Geometry check sheet. Reference: drawing and pictorial views, mm from the part's lowest x, y, z. A direction names the side the tool comes from. Coordinates: 2 decimals unless noted, no trailing zeros. Loops run counter-clockwise (first coordinate to the right, second up) from the corner with the lowest first, then second, coordinate; pieces in that order, holes last. Notation, with made-up numbers: (60, 58.25) - (95, 58.25) arc R30 cw to (95, 83.25) - close; hole circle Ø4 at (12, 48.25). An arc over 180 degrees is marked (long way). One line per item, written item: value.
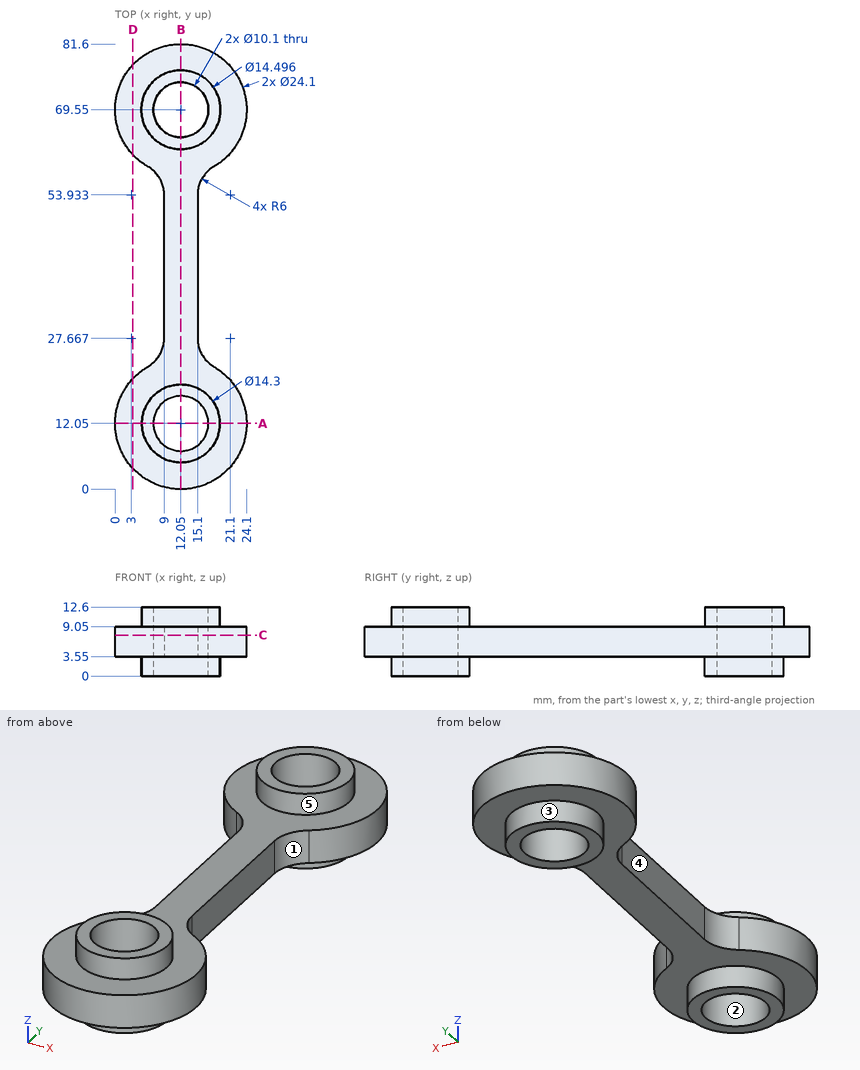
(1) Access from +Z, -Z, +X, -X, +Y, -Y to the whole of each face (thin tool, end or side, straight path). Record for the marked faces 1, 2, 3, 4 and 5.
Reply:
face 1: +Z, -Z, +X
face 2: +Z, -Z
face 3: -Z
face 4: +Z, -Z, -X
face 5: +Z
(2) Cross-section at B-B on x = 12.05. Record the cut outline in (y, z), and give its area (3 significant figures).
Reply:
outline: (0, 3.55) - (4.9, 3.55) - (4.9, 0) - (7, 0) - (7, 12.6) - (4.9, 12.6) - (4.9, 9.05) - (0, 9.05) - close; (17.1, 0) - (19.2, 0) - (19.2, 3.55) - (62.3, 3.55) - (62.3, 0) - (64.5, 0) - (64.5, 12.6) - (62.3, 12.6) - (62.3, 9.05) - (19.2, 9.05) - (19.2, 12.6) - (17.1, 12.6) - close; (74.6, 0) - (76.8, 0) - (76.8, 3.55) - (81.6, 3.55) - (81.6, 9.05) - (76.8, 9.05) - (76.8, 12.6) - (74.6, 12.6) - close
area: 399 mm2
(3) Cross-section at C-C on z = 7.5. Record the cut outline in (x, y), and give its area (3 significant figures).
Reply:
outline: (6.01, 22.48) arc R12.05 ccw (long way) to (18.09, 22.48) arc R6 cw to (15.1, 27.67) - (15.1, 53.93) arc R6 cw to (18.09, 59.12) arc R12.05 ccw (long way) to (6.01, 59.12) arc R6 cw to (9, 53.93) - (9, 27.67) arc R6 cw to start; hole circle Ø10.1 at (12.05, 12.05); hole circle Ø10.1 at (12.05, 69.55)
area: 967 mm2
(4) Material ranges on probe 1 along Y at (x, z) = (12.05, 9.5); probe 2 along Y at (x, z) = (12.05, 5.5); probe 3 along Y at (x, z) = (11, 7) (1 decimal), recorded low to high. Write a range as from..to.
Reply:
probe 1: 4.9..7, 17.1..19.2, 62.3..64.5, 74.6..76.8
probe 2: 0..7, 17.1..64.5, 74.6..81.6
probe 3: 0..7.1, 17..64.6, 74.5..81.6
(5) Cross-section at A-A on y = 12.05. Record the cut outline in (x, z).
Reply:
outline: (0, 3.55) - (4.9, 3.55) - (4.9, 0) - (7, 0) - (7, 12.6) - (4.9, 12.6) - (4.9, 9.05) - (0, 9.05) - close; (17.1, 0) - (19.2, 0) - (19.2, 3.55) - (24.1, 3.55) - (24.1, 9.05) - (19.2, 9.05) - (19.2, 12.6) - (17.1, 12.6) - close
(6) Go/stop test with flat-tipped pins: pin 1 Ø6 at (y, z) = (37.5, 7) entering from +X; pin 2 Ø6 at (y, z) = (70, 9.5) entering from +X; pin 3 Ø3 at (x, z) = (20.5, 6.5) entering from -Y (1 decimal); pin 4 Ø3 at (x, y) = (15, 28) entering from -Z. Record where each tip stops, or that it passes through.
Reply:
pin 1: x = 15.1
pin 2: x = 24.1
pin 3: y = 2.2
pin 4: z = 3.55
(7) Cross-section at D-D on x = 3.25. Record the cut outline in (y, z), and give its area (3 significant figures).
Reply:
outline: (3.82, 3.55) - (20.28, 3.55) - (20.28, 9.05) - (3.82, 9.05) - close; (61.32, 3.55) - (77.78, 3.55) - (77.78, 9.05) - (61.32, 9.05) - close
area: 181 mm2
